The drawing under review shows one solid part. Ordinate dimensions are in mm from its lowest x, y, z. A direction names the side the tool comes from. Round coordinates to 2 decimals unless told otherwise and drop trailing zeros. Write each loop counter-clockwise with the first axis right and the second up, starting at its lowest first coordinate (ties: lowest second). Pieces come first, ordered by that corner, then holes.
Item 1: Machinability: for the marked faces 1 and 2, which of the approach directions +Z, -Z, +X, -X, +Y, -Y give a long, thin tool a straight path to every point of the face, cutting with its end or side? Answer none if there is none.
Item 2: To check wall thickness, follow L1, parallel to Y at x = 10, z = 21.1; L2, parallel to Z at x = 6, y = 3.5; L3, parallel to Y at x = 120.5, z = 10. State the ranges of each line that lie inside material, in increasing order.
Item 3: Add section D-D (x = 59.5). Give the boundary of the cut face in (y, z).
Item 4: Add section B-B (y = 7). Give the boundary of the cut face in (x, z).
Item 5: Clearance check with flat-ended pins moving along their axes: pin 1 Ø1 at (y, z) = (3, 11.5) entering from -X; pin 2 Ø6 at (x, z) = (91.5, 8) entering from +Y; pin 3 Ø5 at (x, y) = (130, 7) entering from -Z. State where each tip first meets the part, or that it passes through.
Item 6: Add section C-C (z = 8.75). Give the boundary of the cut face in (x, y).
Item 7: Add section A-A (x = 130). Give the boundary of the cut face in (y, z).
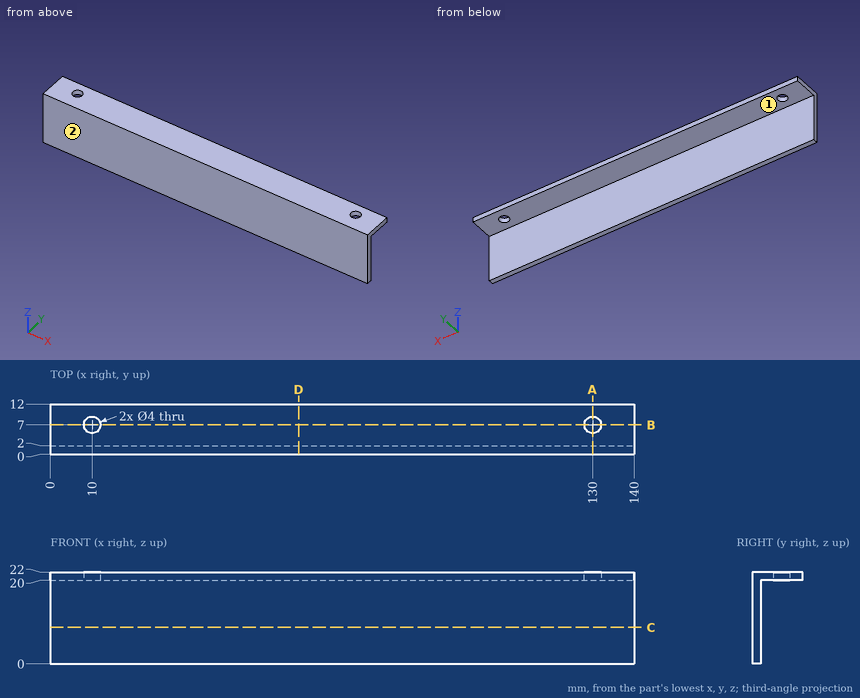
Numbers:
1. face 1: -Z, +X, -X, +Y
1. face 2: +Z, -Z, +X, -X, -Y
2. L1: y = 0 to 5, 9 to 12
2. L2: z = 20 to 22
2. L3: y = 0 to 2
3. outline: (0, 0) - (2, 0) - (2, 20) - (12, 20) - (12, 22) - (0, 22) - close
4. outline: (0, 20) - (8, 20) - (8, 22) - (0, 22) - close; (12, 20) - (128, 20) - (128, 22) - (12, 22) - close; (132, 20) - (140, 20) - (140, 22) - (132, 22) - close
5. pin 1: passes through
5. pin 2: stops at y = 2
5. pin 3: stops at z = 20
6. outline: (0, 0) - (140, 0) - (140, 2) - (0, 2) - close
7. outline: (0, 0) - (2, 0) - (2, 20) - (5, 20) - (5, 22) - (0, 22) - close; (9, 20) - (12, 20) - (12, 22) - (9, 22) - close
